Geometry check sheet. Reference: the model listing, model coordinates, mm. Round coordinates to 2 decimals unless told otherwise and drop trailing zeros. Write each loop counter-clockwise with the first axis right and the second up, starting at its lowest first coordinate (ties: lowest second). Pieces come first, ordered by that corner, then holes.
from build123d import *

# Parameters (mm, degrees)
SKETCH002_R             = 2.6
PAD001_DEPTH            = 2
PAD002_DEPTH            = 2
POCKET003_DEPTH         = 2.201
PAD003_DEPTH            = 2.2
POCKET004_DEPTH         = 4.001
SKETCH006_R             = 17.1
SKETCH006_R_2           = 14.9
POCKET002_DEPTH         = 1
CHAMFER002_SIZE         = 0.4
CHAMFER_SIZE            = 1.99
SKETCH004_R             = 2.2
POCKET_DEPTH            = 4.001
SKETCH005_R             = 6.2
POCKET001_DEPTH         = 2.001
SKETCH010_R             = 4
POCKET005_DEPTH         = 1
CHAMFER001_SIZE         = 1.7
BODY003_PLACEMENT_ANGLE = 240


with BuildPart() as part:
    # Sketch002 → Pad001 (new body)
    with BuildSketch(Plane.XY):
        Polygon((-116.824546, 67.621888), (-37.5, 205.016032), (37.5, 205.016032), (116.824546, 67.621888), (0, 0.173205), align=None)
        with Locations((-51.370835, 167.991041)):
            Circle(SKETCH002_R, mode=Mode.SUBTRACT)
        with Locations((51.370835, 167.991041)):
            Circle(SKETCH002_R, mode=Mode.SUBTRACT)
    extrude(amount=PAD001_DEPTH)

    # Sketch003 → Pad002 (join)
    with BuildSketch(Plane.XY.offset(2)):
        Polygon((-118.899546, 64.027883), (-114.899546, 70.956086), (-0.173205, 4.718802), (-0.173205, 0.1), (-4.173205, -2.209401), align=None)
    extrude(amount=PAD002_DEPTH)

    # Sketch007 → Pocket003 (cut, through all)
    with BuildSketch(Plane.XY.offset(2.2)):
        Polygon((-116.824546, 67.621888), (0, 0.173205), (-4.173205, -2.209401), (-118.899546, 64.027883), align=None)
    extrude(amount=-POCKET003_DEPTH, mode=Mode.SUBTRACT)

    # Sketch008 → Pad003 (join)
    with BuildSketch(Plane.XY):
        Polygon((-104.909165, 58.259933), (-87.588657, 48.259933), (-88.588657, 46.527883), (-105.909165, 56.527883), align=None)
    extrude(amount=PAD003_DEPTH)

    # Sketch009 → Pocket004 (cut, through all)
    with BuildSketch(Plane.XY):
        Polygon((83.830836, 53.168669), (84.960836, 51.211452), (103.666985, 62.011452), (102.536985, 63.968669), align=None)
    extrude(amount=POCKET004_DEPTH, mode=Mode.SUBTRACT)

    # Sketch006 → Pocket002 (cut)
    with BuildSketch(Plane.XY):
        Circle(SKETCH006_R)
        Circle(SKETCH006_R_2, mode=Mode.SUBTRACT)
    extrude(amount=POCKET002_DEPTH, mode=Mode.SUBTRACT)

    # Chamfer002
    chamfer002_edges = [part.edges().sort_by_distance(p)[0] for p in [
        (-96.248911, 53.259933, 0),
        (-88.088657, 47.393908, 0),
        (-97.248911, 51.527883, 0),
        (-105.409165, 57.393908, 0),
        (94.313911, 56.611452, 0),
        (103.101985, 62.99006, 0),
        (93.183911, 58.568669, 0),
        (84.395836, 52.19006, 0),
        (0, 14.9, 0),
        (0, 17.1, 0),
    ]]
    chamfer(chamfer002_edges, length=CHAMFER002_SIZE)

    # Chamfer
    chamfer_edges = [part.edges().sort_by_distance(p)[0] for p in [
        (-57.536375, 37.837444, 4),
    ]]
    chamfer(chamfer_edges, length=CHAMFER_SIZE)

    # Sketch004 → Pocket (cut, through all)
    with BuildSketch(Plane.XY):
        Circle(SKETCH004_R)
    extrude(amount=POCKET_DEPTH, mode=Mode.SUBTRACT)

    # Sketch005 → Pocket001 (cut, through all)
    with BuildSketch(Plane.XY.offset(2)):
        Circle(SKETCH005_R)
    extrude(amount=POCKET001_DEPTH, mode=Mode.SUBTRACT)

    # Sketch010 → Pocket005 (cut)
    with BuildSketch(Plane.XY.offset(2)):
        with Locations((-51.370835, 167.991041)):
            Circle(SKETCH010_R)
        with Locations((51.370835, 167.991041)):
            Circle(SKETCH010_R)
    extrude(amount=-POCKET005_DEPTH, mode=Mode.SUBTRACT)

    # Chamfer001
    chamfer001_edges = [part.edges().sort_by_distance(p)[0] for p in [
        (-5.849077, 2.056283, 4),
        (-62.500992, 31.466162, 4),
        (-117.397046, 66.630289, 4),
    ]]
    chamfer(chamfer001_edges, length=CHAMFER001_SIZE)


with BuildPart() as part_1:
    # Body003 placement: moved
    add(part.part.rotate(Axis((0, 0, 0), (0, 0, 1)), BODY003_PLACEMENT_ANGLE))


solid = part_1.part
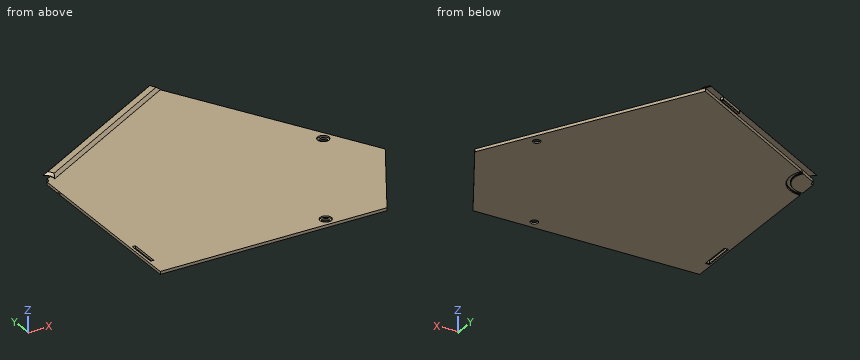
1. Scan lines: line 1 along X through (y, z) = (-113, 0.45); line 2 along Z through (x, y) = (131, -11); line 3 along X through (y, z) = (-107.5, 1.7). Record each from-to range of solid material in increasing order.
2. Section check D-D (z = 3). Record the cut outline in (x, y), plus the area to 3 significant figures.
3. Depth check by flat-ended pin: pin 1 Ø4 at (x, y) = (169.5, -39) entering from +Z; pin 2 Ø6.5 at (x, y) = (119, -126.5) entering from +Z; pin 3 Ø5 at (x, y) = (119.8, -128.48) entering from +Z; pin 4 Ø18.5 at (x, y) = (10, -1.5) entering from -Z. Enter the tip coordinate at first touch or a pass-through.
Results below:
1. line 1: x = 0.15 to 1.87, 4.13 to 171.49
1. line 2: z = 0 to 2
1. line 3: x = 0.15 to 1.87, 4.13 to 174.67
2. outline: (3.6, 5.89) arc R6.9 cw to (6.88, 0.5) - (117.8, 64.54) - (114.64, 70) - close
2. area: 805 mm2
3. pin 1: stops at z = 1
3. pin 2: stops at z = 2
3. pin 3: passes through
3. pin 4: stops at z = 0
